```python
from build123d import *

# Parameters (mm, degrees)
BOSS_EXTRUDE1_DEPTH = 7.5
SKETCH2_R           = 2.5
BOSS_EXTRUDE2_DEPTH = 20
SKETCH3_R           = 7.5
CUT_EXTRUDE1_DEPTH  = 271.257400454
CUT_EXTRUDE2_DEPTH  = 20


with BuildPart() as part:
    # Sketch1 → Boss-Extrude1 (new body)
    with BuildSketch(Plane(origin=(0, 0, 0), x_dir=(1, 0, 0), z_dir=(0, 1, 0))):
        Polygon((0, 0), (-150, 0), (-150, -55), (-150, -155), (-150, -210), (0, -210), align=None)
    extrude(amount=BOSS_EXTRUDE1_DEPTH)

    # Sketch2 → Boss-Extrude2 (add)
    with BuildSketch(Plane.ZY.offset(150)):
        with BuildLine():
            Line((205, 6.25), (5, 6.25))
            ThreePointArc((5, 6.25), (6.767766953, 5.517766953), (7.5, 3.75))
            ThreePointArc((7.5, 3.75), (6.767766953, 1.982233047), (5, 1.25))
            Line((5, 1.25), (205, 1.25))
            ThreePointArc((205, 1.25), (202.5, 3.75), (205, 6.25))
        make_face()
        with Locations((205, 3.75)):
            Circle(SKETCH2_R)
        with Locations((5, 3.75)):
            Circle(SKETCH2_R)
    extrude(amount=BOSS_EXTRUDE2_DEPTH)

    # Sketch3 → Cut-Extrude1 (cut, through all)
    with BuildSketch(Plane(origin=(0, 6.25, 0), x_dir=(1, 0, 0), z_dir=(0, 1, 0))):
        with BuildLine():
            ThreePointArc((-152.5, -15), (-160, -22.5), (-167.5, -15))
            Line((-167.5, -15), (-167.5, -195))
            ThreePointArc((-167.5, -195), (-160, -187.5), (-152.5, -195))
            Line((-152.5, -195), (-152.5, -15))
        make_face()
        with Locations((-160, -15)):
            Circle(SKETCH3_R)
        with Locations((-160, -195)):
            Circle(SKETCH3_R)
    extrude(amount=-CUT_EXTRUDE1_DEPTH, mode=Mode.SUBTRACT)

    # Sketch4 → Cut-Extrude2 (cut)
    with BuildSketch(Plane(origin=(0, 6.25, 0), x_dir=(1, 0, 0), z_dir=(0, 1, 0))):
        with BuildLine():
            ThreePointArc((-166.614378278, -5), (-163.535533906, -3.145856533), (-160, -2.5))
            Line((-160, -2.5), (-170, -2.5))
            Line((-170, -2.5), (-170, -5))
            Line((-170, -5), (-166.614378278, -5))
        make_face()
        with BuildLine():
            ThreePointArc((-170, -12.5), (-169.114378278, -8.385621722), (-166.614378278, -5))
            Line((-166.614378278, -5), (-170, -5))
            Line((-170, -5), (-170, -12.5))
        make_face()
        with BuildLine():
            ThreePointArc((-160, -207.5), (-163.535533906, -206.854143467), (-166.614378278, -205))
            Line((-166.614378278, -205), (-170, -205))
            Line((-170, -205), (-170, -207.5))
            Line((-170, -207.5), (-160, -207.5))
        make_face()
        with BuildLine():
            Line((-170, -205), (-166.614378278, -205))
            ThreePointArc((-166.614378278, -205), (-169.114378278, -201.614378278), (-170, -197.5))
            Line((-170, -197.5), (-170, -205))
        make_face()
    extrude(amount=-CUT_EXTRUDE2_DEPTH, mode=Mode.SUBTRACT)


solid = part.part
```
Part model, mm, in its own coordinate system. A direction names the side the tool comes from. Round coordinates to 2 decimals unless told otherwise and drop trailing zeros. Write each loop counter-clockwise with the first axis right and the second up, starting at its lowest first coordinate (ties: lowest second). Pieces come first, ordered by that corner, then holes. Notation, with made-up numbers: M -20,16 L 23,16 A17 ccw 23,28 Z; hole C 76.5,22.25 d1. An arc over 180 degrees is marked long. Answer as CSV lines item,"result". Start each with the question number.
1) Band-saw the part on B-B (y = 3.75). List the corners of the cut face in (x, z), then the cut area to 3 significant figures.
2) Which spindle directions (+Z, -Z, +X, -X, +Y, -Y) get a long thin tool onto all of the face, cutting with end or side? Do faces 1 (the face through (-156.3, 3.7, 207.5)), 2 (the face through (-152, 6.25, 105)), 3 (the face through (-167.5, 4, 104)), 4 (the face through (-74, 4, 0)). Say none if no direction does.
3) Mould opens along Z. For faces 5 (the face through (-152, 1.25, 105)), 6 (the face through (-152.5, 4, 106)), 7 (the face through (-156.3, 3.8, 2.5)) say: +Z half, -Z half, draft (parallel to the pull), parting line (faces both ways), or undercut.
4) Band-saw the part on A-A (z = 68). List the corners of the cut face in (x, y).
5) Drop a flat-ended pin along its axis: pin 1 (22 mm diameter, centred on x = -164, z = 145, fed in from +Y). Give the stop position or say it passes through.
6) Drill centre lines: L1, parallel to X at y = 2.75, z = 93; L2, parallel to X at y = 1, z = 113; L3, parallel to Z at x = -159.5, y = 4.5. Where is each one in solid material? Low to high.
Worked out:
1,outline,"M -170,12.5 A10 ccw -160,2.5 L -150,2.5 L -150,0 L 0,0 L 0,210 L -150,210 L -150,207.5 L -160,207.5 A10 ccw -170,197.5 Z; hole M -167.5,15 A7.5 ccw -152.5,15 L -152.5,195 A7.5 ccw -167.5,195 Z"
1,area,"32,700 mm²"
2,face 1,"+Z, -X"
2,face 2,"+Z, -Z, -X, +Y"
2,face 3,"+Y, -Y"
2,face 4,"-Z, +X, -X, +Y, -Y"
3,face 5,"draft"
3,face 6,"undercut"
3,face 7,"-Z half"
4,outline,"M -170,1.25 L -167.5,1.25 L -167.5,6.25 L -170,6.25 Z; M -152.5,1.25 L -150,1.25 L -150,0 L 0,0 L 0,7.5 L -150,7.5 L -150,6.25 L -152.5,6.25 Z"
5,pin 1,"y = 6.25"
6,L1,"-170 to -167.5, -152.5 to 0"
6,L2,"-150 to 0"
6,L3,"2.62 to 7.52, 202.48 to 207.38"
